```python
from build123d import *


with BuildPart() as part:
    # Esquisse1 → Base-Révolution (revolve)
    with BuildSketch(Plane.XY, mode=Mode.PRIVATE) as base_r_volution_sk:
        with BuildLine():
            Line((6.2, 0), (9, 0))
            Line((9, 0), (9, 1))
            Line((9, 1), (6.2, 1))
            ThreePointArc((6.2, 1), (6.058578644, 1.058578644), (6, 1.2))
            Line((6, 1.2), (6, 6.8))
            ThreePointArc((6, 6.8), (6.058578644, 6.941421356), (6.2, 7))
            Line((6.2, 7), (9, 7))
            Line((9, 7), (9, 8))
            Line((9, 8), (6.2, 8))
            ThreePointArc((6.2, 8), (5.351471863, 7.648528137), (5, 6.8))
            Line((5, 6.8), (5, 1.2))
            ThreePointArc((5, 1.2), (5.351471863, 0.351471863), (6.2, 0))
        make_face()
    revolve(base_r_volution_sk.sketch.rotate(Axis((0, 0, 0), (0, 1, 0)), 90), axis=Axis((0, 0, 0), (0, 1, 0)))


solid = part.part
```
Build history of the part. All positions in model axes, mm. A direction names the side the tool comes from. Coordinates: 2 decimals unless noted, no trailing zeros. Order: outer loops, then holes, each group sorted by start corner. A loop starts at its lowest first (then second) coordinate and runs counter-clockwise, first axis right, second up. Notation, with made-up numbers: (47, 80) -> (65, 80) arc R22 ccw to (65, 86) -> close; hole circle Ø8 at (47, -31). An arc over 180 degrees is marked (long way). Answer in a Markdown table with one row per item. Add a question column.
Q1. Band-saw the part on A-A, the plane x = 0. List the corners of the cut face in (y, z).
Q2. Which spindle directions (+Z, -Z, +X, -X, +Y, -Y) get a long thin tool onto all of the face, cutting with end or side? Do faces 1 (the face through (1.9, 0, -6.1)), 2 (the face through (1.9, 1, 6.1)). Say none if no direction does.
Q3. Wall check: line 1 along X through (y, z) = (4.1, 0); line 2 along Y through (x, z) = (-5.75, -5.25); line 3 along X through (y, z) = (6.5, -1.5). Give the ranges that are in metal, low to high. Write a range as [from, to].
Q4. Band-saw the part on B-B, the plane z = 0. List the corners of the cut face in (x, y).
Q5. Mould opens along Z. For faces 3 (the face through (1.9, 8, 6.1)), 4 (the face through (-6.083, 7.507, 6.633)), 5 (the face through (0, 4, 5)) say: +Z half, -Z half, draft (parallel to the pull), parting line (faces both ways), or undercut.
Q6. Band-saw the part on D-D, the plane z = -6.5. List the corners of the cut face in (x, y).
Q7. Band-saw the part on C-C, the plane y = 6. List the corners of the cut face in (x, z), then the cut area to 3 significant figures.
Q8. Drop flat-ended pins along their axis: pin 1 (4 mm diameter, centred on x = 2.5, z = -1, fed in from -Y); pin 2 (1.5 mm diameter, centred on x = 2.5, y = 5, fed in from +Z); pin 3 (4 mm diameter, centred on y = 2, z = -5, fed in from -X). Give the stop position or say it passes through.
Answers follow:
| question | item | result |
|---|---|---|
| 1 | outline | (0, -9) -> (1, -9) -> (1, -6.2) arc R0.2 cw to (1.2, -6) -> (6.8, -6) arc R0.2 cw to (7, -6.2) -> (7, -9) -> (8, -9) -> (8, -6.2) arc R1.2 ccw to (6.8, -5) -> (1.2, -5) arc R1.2 ccw to (0, -6.2) -> close; (0, 6.2) arc R1.2 ccw to (1.2, 5) -> (6.8, 5) arc R1.2 ccw to (8, 6.2) -> (8, 9) -> (7, 9) -> (7, 6.2) arc R0.2 cw to (6.8, 6) -> (1.2, 6) arc R0.2 cw to (1, 6.2) -> (1, 9) -> (0, 9) -> close |
| 2 | face 1 | +Z, -Z, +X, -X, -Y |
| 2 | face 2 | none |
| 3 | line 1 | [-6, -5], [5, 6] |
| 3 | line 2 | [0, 1], [7, 8] |
| 3 | line 3 | [-5.81, -4.77], [4.77, 5.81] |
| 4 | outline | (-9, 0) -> (-6.2, 0) arc R1.2 ccw to (-5, 1.2) -> (-5, 6.8) arc R1.2 ccw to (-6.2, 8) -> (-9, 8) -> (-9, 7) -> (-6.2, 7) arc R0.2 cw to (-6, 6.8) -> (-6, 1.2) arc R0.2 cw to (-6.2, 1) -> (-9, 1) -> close; (5, 1.2) arc R1.2 ccw to (6.2, 0) -> (9, 0) -> (9, 1) -> (6.2, 1) arc R0.2 cw to (6, 1.2) -> (6, 6.8) arc R0.2 cw to (6.2, 7) -> (9, 7) -> (9, 8) -> (6.2, 8) arc R1.2 ccw to (5, 6.8) -> close |
| 5 | face 3 | draft |
| 5 | face 4 | parting line |
| 5 | face 5 | undercut |
| 6 | outline | (-6.22, 0) -> (6.22, 0) -> (6.22, 1) -> (-6.22, 1) -> close; (-6.22, 7) -> (6.22, 7) -> (6.22, 8) -> (-6.22, 8) -> close |
| 7 | outline | circle Ø12 at (0, 0); hole circle Ø10 at (0, 0) |
| 7 | area | 34.6 mm^2 |
| 8 | pin 1 | through |
| 8 | pin 2 | z = 5.74 |
| 8 | pin 3 | x = -8.39 |
